Check sheet for the modelled part. Datum: model origin and axes. Units: mm. A direction names the side the tool comes from. Coordinates: 2 decimals unless noted, no trailing zeros. Order: outer loops, then holes, each group sorted by start corner. A loop starts at its lowest first (then second) coordinate and runs counter-clockwise, first axis right, second up.
1. Set-up check for faces 1 (the flat face through (-1, -4, 4)), 2 (the cylindrical face through (9.139, 14.334, 48.684)), 3 (the flat face through (7, -14, 44)), 4 (the flat face through (15, -13.44, 4)), 5 (the flat face through (3, 7, 0)): record each of +Z, -Z, +X, -X, +Y, -Y from which the full face is reachable in a straight line by a thin tool's end or side.
2. Cross-section at B-B (z = 65.5). Enter the section's corners in (x, y).
3. Gauge pin test, flat ends, axial feed: pin 1 Ø18 at (x, y) = (0, 0) entering from +Z; pin 2 Ø6.5 at (x, z) = (16, 2.5) entering from -Y; pin 3 Ø10 at (x, y) = (-7.5, 0.5) entering from +Z. Record the tip position at first contact, or that the pin passes through.
4. Thickness scan on line 1 (Z direction, x = 2.5, y = -16.5); line 2 (Y direction, x = 0, z = 77.5); line 3 (Z direction, x = 13, y = -2.5). Record the ranges inside material, lowest first.
5. Draft check along X on faces 6 (the flat face through (19, 0, 19)), 7 (the flat face through (0, 19, 19)), 8 (the cylindrical face through (8.06, -12.65, 78.47)), 9 (the flat face through (-5, -10, 76.5)). Enter one of: released by +X, released by -X, zero draft, split by the parting line, or undercut.
```python
from build123d import *

# Parameters (mm, degrees)
SKETCH_1_W          = 38
SKETCH_1_H          = 38
EXTRUDE_1_DEPTH     = 38
SKETCH_2_R          = 15.5
EXTRUDE_2_DEPTH     = 6
SKETCH_3_R          = 17
EXTRUDE_3_DEPTH     = 9.5
SKETCH_4_R          = 16.5
EXTRUDE_4_DEPTH     = 7.5
SKETCH_5_R          = 17
EXTRUDE_5_DEPTH     = 7.5
SKETCH_6_R          = 16.5
EXTRUDE_6_DEPTH     = 12
CUT_EXTRUDE_1_DEPTH = 9


with BuildPart() as part:
    # 草图1 → 拉伸1 (new body)
    with BuildSketch(Plane.XY):
        Rectangle(SKETCH_1_W, SKETCH_1_H)
    extrude(amount=EXTRUDE_1_DEPTH)

    # 草图2 → 拉伸2 (add)
    with BuildSketch(Plane.XY.offset(38)):
        Circle(SKETCH_2_R)
    extrude(amount=EXTRUDE_2_DEPTH)

    # 草图3 → 拉伸3 (add)
    with BuildSketch(Plane.XY.offset(44)):
        Circle(SKETCH_3_R)
    extrude(amount=EXTRUDE_3_DEPTH)

    # 草图4 → 拉伸4 (add)
    with BuildSketch(Plane.XY.offset(53.5)):
        Circle(SKETCH_4_R)
    extrude(amount=EXTRUDE_4_DEPTH)

    # 草图5 → 拉伸5 (add)
    with BuildSketch(Plane.XY.offset(61)):
        Circle(SKETCH_5_R)
    extrude(amount=EXTRUDE_5_DEPTH)

    # 草图6 → 拉伸6 (add)
    with BuildSketch(Plane.XY.offset(68.5)):
        Circle(SKETCH_6_R)
    extrude(amount=EXTRUDE_6_DEPTH)

    # 草图8 → 切除-旋转1 (revolve, cut)
    with BuildSketch(Plane(origin=(0, 0, 0), x_dir=(1, 0, 0), z_dir=(0, 1, 0)), mode=Mode.PRIVATE) as cut_revolve_1_sk:
        with BuildLine():
            Line((0, -80.5), (-15, -80.5))
            Line((-15, -80.5), (-15, -76.5))
            Line((-15, -76.5), (-11, -76.5))
            Line((-11, -76.5), (-9.5, -73.5))
            ThreePointArc((-9.5, -73.5), (-4.842577395, -74.909003343), (0, -75.384734276))
            Line((0, -75.384734276), (0, -80.5))
        make_face()
    revolve(cut_revolve_1_sk.sketch.rotate(Axis((0, 0, 1080.5), (0, 0, -1)), 180), axis=Axis((0, 0, 1080.5), (0, 0, -1)), mode=Mode.SUBTRACT)

    # 草图9 → 切除-拉伸1 (cut)
    with BuildSketch(Plane(origin=(0, 0, 0), x_dir=(-1, 0, 0), z_dir=(0, 0, -1))):
        Polygon((-19, -19), (19, -19), (19, 19), (13, 19), (13, -4), (-11, -4), (-11, -13.44), (-19, -13.44), align=None)
    extrude(amount=-CUT_EXTRUDE_1_DEPTH, mode=Mode.SUBTRACT)


solid = part.part
```
Data:
1. face 1: -Z, -X, -Y
1. face 2: +Z
1. face 3: none
1. face 4: -Z, +X, -X, -Y
1. face 5: -Z, +X, -X, +Y, -Y
2. outline: circle Ø34 at (0, 0)
3. pin 1: stops at z = 75.38
3. pin 2: stops at y = -13.44
3. pin 3: stops at z = 76.5
4. line 1: z = 9 to 38, 44 to 53.5, 61 to 68.5
4. line 2: y = -16.5 to -15, 15 to 16.5
4. line 3: z = 0 to 76.5
5. face 6: released by +X
5. face 7: zero draft
5. face 8: undercut
5. face 9: undercut
